Geometry check sheet. Reference: drawing and pictorial views, mm from the part's lowest x, y, z. Round coordinates to 2 decimals unless told otherwise and drop trailing zeros. Write each loop counter-clockwise with the first axis right and the second up, starting at its lowest first coordinate (ties: lowest second). Pieces come first, ordered by that corner, then holes. Notation, with made-up numbers: M -24.5,23 L -19.5,23 A13 ccw -19.5,37 Z; hole C 62,-5 d2. An arc over 180 degrees is marked long. Put each result on its own line as item: value. Start each with the question number.
(1) Section check A-A on y = 24. Record the cut outline in (x, z) (3 decimals), then the cut area to 3 significant figures.
(2) Section check B-B on z = 2.55. Record the cut outline in (x, y).
(3) Gauge pin test, flat end, axial feed: pin 1 (3.5 mm diameter, centred on x = 12.7, y = 38.1, fed in from -Z). Record the tip position at first contact, or that the pin passes through.
(4) Material ranges on probe 1 along Y at (x, z) = (12.7, 1.1); probe 2 along X at (y, z) = (30, 2.9); probe 3 along X at (y, z) = (39, 3) (1 decimal), recorded low to high.
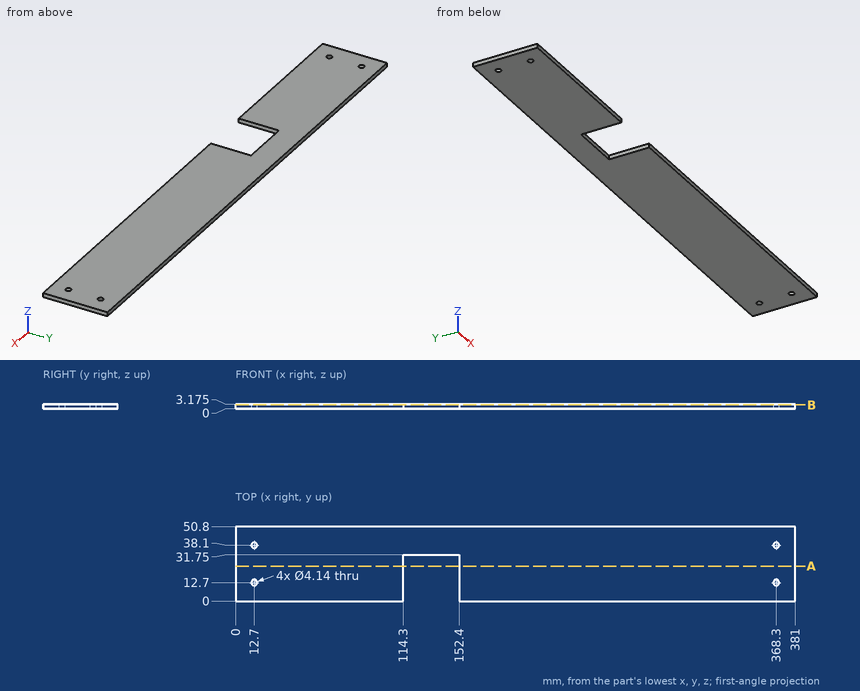
Answers follow:
1. outline: M 0,0 L 114.3,0 L 114.3,3.175 L 0,3.175 Z; M 152.4,0 L 381,0 L 381,3.175 L 152.4,3.175 Z
1. area: 1,090 mm^2
2. outline: M 0,0 L 114.3,0 L 114.3,31.75 L 152.4,31.75 L 152.4,0 L 381,0 L 381,50.8 L 0,50.8 Z; hole C 12.7,12.7 d4.14; hole C 12.7,38.1 d4.14; hole C 368.3,12.7 d4.14; hole C 368.3,38.1 d4.14
3. pin 1: passes through
4. probe 1: y = 0 to 10.63, 14.77 to 36.03, 40.17 to 50.8
4. probe 2: x = 0 to 114.3, 152.4 to 381
4. probe 3: x = 0 to 10.8, 14.6 to 366.4, 370.2 to 381
